Part print with two shaded views. Sizes in mm from the minimum x, y, z corner. Round coordinates to 2 decimals unless told otherwise and drop trailing zeros. Order: outer loops, then holes, each group sorted by start corner. A loop starts at its lowest first (then second) coordinate and runs counter-clockwise, first axis right, second up. Notation, with made-up numbers: (40, 29) -> (62, 29) arc R20 cw to (62, 39) -> close; hole circle Ø3 at (20.25, -14). An arc over 180 degrees is marked (long way). Answer as a JSON object with one key per item and string values.
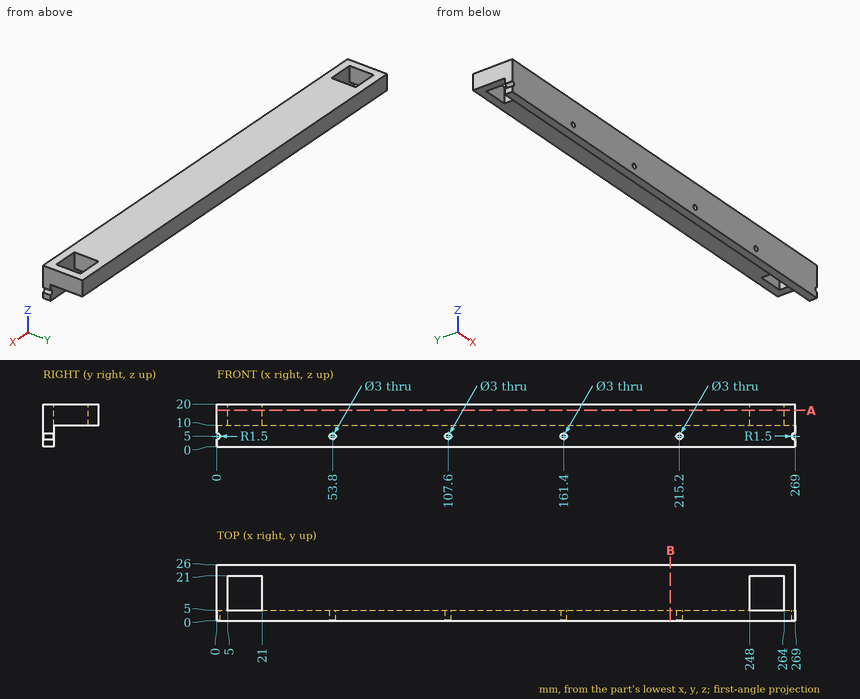
1) Cut at B-B, the plane x = 211. Give the cut face in (y, z), plus the area to 3 significant figures.
Checked values:
{"outline": "(0, 0) -> (5, 0) -> (5, 10) -> (26, 10) -> (26, 20) -> (0, 20) -> close", "area": "310 mm²"}
2) Probe L1, parallel to Z at x = 107.6, y = 1.6; L2, parallel to Z at x = 188, y = 18.25; L3, parallel to Y at x = 163.5, z = 4. List the from-to ranges inside material, lowest first. Write a range as from..to.
Checked values:
{"L1": "z = 0..3.5, 6.5..20", "L2": "z = 10..20", "L3": "y = 0..5"}
3) Flat gauge pins, fed straight in: pin 1 Ø4 at (x, z) = (215.2, 5) entering from +Y; pin 2 Ø12 at (y, z) = (10, 12) entering from -X; pin 3 Ø12 at (x, y) = (65, 17.5) entering from -Z. Where does each tip first touch, or does it go through?
Checked values:
{"pin 1": "stops at y = 5", "pin 2": "stops at x = 0", "pin 3": "stops at z = 10"}
4) Cut at A-A, the plane z = 17. Give the cut face in (x, y), plus the area to 3 significant figures.
Checked values:
{"outline": "(0, 0) -> (269, 0) -> (269, 26) -> (0, 26) -> close; hole (5, 5) -> (21, 5) -> (21, 21) -> (5, 21) -> close; hole (248, 5) -> (264, 5) -> (264, 21) -> (248, 21) -> close", "area": "6,480 mm²"}
